from build123d import *

# Parameters (mm, degrees)
SKETCH1_R           = 15
BOSS_EXTRUDE1_DEPTH = 7.5
SKETCH2_R           = 7.90082564
BOSS_EXTRUDE2_DEPTH = 10


with BuildPart() as part:
    # Sketch1 → Boss-Extrude1 (new body, symmetric)
    with BuildSketch(Plane(origin=(0, 0, 0), x_dir=(1, 0, 0), z_dir=(0, 1, 0))):
        with BuildLine():
            Line((7.75, 99.699235203), (7.75, 63))
            ThreePointArc((7.75, 63), (0, 55.25), (-7.75, 63))
            Line((-7.75, 63), (-7.75, 99.699235203))
            ThreePointArc((-7.75, 99.699235203), (-12.394488334, 99.228910399), (-17.011966007, 98.542341217))
            ThreePointArc((-17.011966007, 98.542341217), (-40, 69.282032303), (-76.834187839, 64.003965339))
            ThreePointArc((-76.834187839, 64.003965339), (-79.737513028, 60.348396964), (-82.467070423, 56.561314481))
            Line((-82.467070423, 56.561314481), (-50.684600438, 38.211696879))
            ThreePointArc((-50.684600438, 38.211696879), (-47.847903559, 35.375), (-46.809600438, 31.5))
            ThreePointArc((-46.809600438, 31.5), (-50.684600438, 24.788303121), (-58.434600438, 24.788303121))
            Line((-58.434600438, 24.788303121), (-90.217070423, 43.137920722))
            ThreePointArc((-90.217070423, 43.137920722), (-92.132001362, 38.880513435), (-93.846153846, 34.538375878))
            ThreePointArc((-93.846153846, 34.538375878), (-80, 0), (-93.846153846, -34.538375878))
            ThreePointArc((-93.846153846, -34.538375878), (-92.132001362, -38.880513435), (-90.217070423, -43.137920722))
            Line((-90.217070423, -43.137920722), (-58.434600438, -24.788303121))
            ThreePointArc((-58.434600438, -24.788303121), (-50.684600438, -24.788303121), (-46.809600438, -31.5))
            ThreePointArc((-46.809600438, -31.5), (-47.847903559, -35.375), (-50.684600438, -38.211696879))
            Line((-50.684600438, -38.211696879), (-82.467070423, -56.561314481))
            ThreePointArc((-82.467070423, -56.561314481), (-79.737513028, -60.348396964), (-76.834187839, -64.003965339))
            ThreePointArc((-76.834187839, -64.003965339), (-40, -69.282032303), (-17.011966007, -98.542341217))
            ThreePointArc((-17.011966007, -98.542341217), (-12.394488334, -99.228910399), (-7.75, -99.699235203))
            Line((-7.75, -99.699235203), (-7.75, -63))
            ThreePointArc((-7.75, -63), (0, -55.25), (7.75, -63))
            Line((7.75, -63), (7.75, -99.699235203))
            ThreePointArc((7.75, -99.699235203), (12.394488334, -99.228910399), (17.011966007, -98.542341217))
            ThreePointArc((17.011966007, -98.542341217), (40, -69.282032303), (76.834187839, -64.003965339))
            ThreePointArc((76.834187839, -64.003965339), (79.737513028, -60.348396964), (82.467070423, -56.561314481))
            Line((82.467070423, -56.561314481), (50.684600438, -38.211696879))
            ThreePointArc((50.684600438, -38.211696879), (47.847903559, -27.625), (58.434600438, -24.788303121))
            Line((58.434600438, -24.788303121), (90.217070423, -43.137920722))
            ThreePointArc((90.217070423, -43.137920722), (92.132001362, -38.880513435), (93.846153846, -34.538375878))
            ThreePointArc((93.846153846, -34.538375878), (80, 0), (93.846153846, 34.538375878))
            ThreePointArc((93.846153846, 34.538375878), (92.132001362, 38.880513435), (90.217070423, 43.137920722))
            Line((90.217070423, 43.137920722), (58.434600438, 24.788303121))
            ThreePointArc((58.434600438, 24.788303121), (47.847903559, 27.625), (50.684600438, 38.211696879))
            Line((50.684600438, 38.211696879), (82.467070423, 56.561314481))
            ThreePointArc((82.467070423, 56.561314481), (79.737513028, 60.348396964), (76.834187839, 64.003965339))
            ThreePointArc((76.834187839, 64.003965339), (40, 69.282032303), (17.011966007, 98.542341217))
            ThreePointArc((17.011966007, 98.542341217), (12.394488334, 99.228910399), (7.75, 99.699235203))
        make_face()
        Circle(SKETCH1_R, mode=Mode.SUBTRACT)
    extrude(amount=BOSS_EXTRUDE1_DEPTH, both=True)

    # Sketch2 → Boss-Extrude2 (add)
    with BuildSketch(Plane(origin=(0, 7.5, 0), x_dir=(1, 0, 0), z_dir=(0, 1, 0))):
        with Locations((33.709720075, 58.386947879)):
            Circle(SKETCH2_R)
        with Locations((67.41944015, 0)):
            Circle(SKETCH2_R)
        with Locations((33.709720075, -58.386947879)):
            Circle(SKETCH2_R)
        with Locations((-33.709720075, -58.386947879)):
            Circle(SKETCH2_R)
        with Locations((-67.41944015, 0)):
            Circle(SKETCH2_R)
        with Locations((-33.709720075, 58.386947879)):
            Circle(SKETCH2_R)
    extrude(amount=BOSS_EXTRUDE2_DEPTH)


solid = part.part
CAD build for the part. Positions are in the model's coordinates, mm. A direction names the side the tool comes from. Round coordinates to 2 decimals unless told otherwise and drop trailing zeros. Write each loop counter-clockwise with the first axis right and the second up, starting at its lowest first coordinate (ties: lowest second). Pieces come first, ordered by that corner, then holes. Notation, with made-up numbers: M 41.5,82.25 L 86.5,82.25 A32 ccw 86.5,116.25 Z; hole C -7,75 d4. An arc over 180 degrees is marked long. Use a Markdown table: item, result. Add a question column.
1. Drill centre lines: probe 1 along X at (y, z) = (-1.25, 34); probe 2 along Z at (x, y) = (-33.5, 13.5); probe 3 along Z at (x, y) = (0, 1). Where is each one in solid material? Low to high.
2. Flat gauge pins, fed straight in: P1, Ø12, axis at y = 2, z = -82.5, coming from the +X side; P2, Ø7.5, axis at y = -2, z = 89, coming from the +X side; P3, Ø4, axis at x = -16, z = -33.5, coming from the +Y side. Where does each tip first touch, or does it go through?
3. 3-axis set-ups, long thin cutter, end or side, ignore diameter. For faces 1 (the face through (7.75, 0, -82)), 2 (the face through (74.718, 12.43, 3.026)), 3 (the face through (-66.798, 0.105, -47.515)), 4 (the face through (-7.75, 0, 82)): which of +Z, -Z, +X, -X, +Y, -Y reach the whole face in a straight line?
4. Slice it at C-C on x = 64. Give the cut face in (y, z), then the cut area to 3 significant figures.
5. Slice it at B-B on z = 0. Give the cut face in (x, y), then the cut area to 3 significant figures.
6. Pull direction X, two halves, no side cores. Call faces 5 (the face through (25.817, 12.43, 58.04)), 6 (the face through (-12.33, 0.105, -99.237)), 7 (the face through (92.157, 0.105, -38.82)), 8 (the face through (74.103, 0.105, 33.835)): released by +X, released by -X, zero draft, split by the parting line, or undercut.
7. Slice it at D-D on z = -72.5. Give the cut face in (x, y).
8. Slice it at A-A on x = 0. Give the cut face in (y, z).
Reply:
| question | item | result |
|---|---|---|
| 1 | probe 1 | x = -93.34 to -74.39, -47.22 to 47.22, 74.39 to 93.34 |
| 1 | probe 2 | z = -66.28 to -50.49, 50.49 to 66.28 |
| 1 | probe 3 | z = -55.25 to -15, 15 to 55.25 |
| 2 | P1 | stops at x = 30.39 |
| 2 | P2 | stops at x = 23.13 |
| 2 | P3 | stops at y = 7.5 |
| 3 | face 1 | -Z, +Y, -Y |
| 3 | face 2 | +Y |
| 3 | face 3 | +Y, -Y |
| 3 | face 4 | +Z, +Y, -Y |
| 4 | outline | M -7.5,-62.59 L 7.5,-62.59 L 7.5,-45.9 L -7.5,-45.9 Z; M -7.5,-28 L 7.5,-28 L 7.5,-7.12 L 17.5,-7.12 L 17.5,7.12 L 7.5,7.12 L 7.5,28 L -7.5,28 Z; M -7.5,45.9 L 7.5,45.9 L 7.5,62.59 L -7.5,62.59 Z |
| 4 | area | 1,480 mm^2 |
| 5 | outline | M -80,-7.5 L -15,-7.5 L -15,7.5 L -59.52,7.5 L -59.52,17.5 L -75.32,17.5 L -75.32,7.5 L -80,7.5 Z; M 15,-7.5 L 80,-7.5 L 80,7.5 L 75.32,7.5 L 75.32,17.5 L 59.52,17.5 L 59.52,7.5 L 15,7.5 Z |
| 5 | area | 2,270 mm^2 |
| 6 | face 5 | undercut |
| 6 | face 6 | released by -X |
| 6 | face 7 | released by +X |
| 6 | face 8 | undercut |
| 7 | outline | M -35.11,-7.5 L -7.75,-7.5 L -7.75,7.5 L -35.11,7.5 Z; M 7.75,-7.5 L 35.11,-7.5 L 35.11,7.5 L 7.75,7.5 Z |
| 8 | outline | M -7.5,-55.25 L 7.5,-55.25 L 7.5,-15 L -7.5,-15 Z; M -7.5,15 L 7.5,15 L 7.5,55.25 L -7.5,55.25 Z |
